Could you check a few things on this model? Use its own coordinates, in mm. A direction names the side the tool comes from. Round coordinates to 2 decimals unless told otherwise and drop trailing zeros. Order: outer loops, then holes, each group sorted by start corner. A loop starts at its lowest first (then second) coordinate and runs counter-clockwise, first axis right, second up. Notation, with made-up numbers: (85, 88) -> (110, 88) arc R26 cw to (110, 104) -> close; hole circle Ø5 at (-1.5, -28). An arc over 180 degrees is marked (long way). One line per question, with ' | ' between items.
```python
from build123d import *

# Parameters (mm, degrees)
CROQUIS1_R              = 2
SALIENTE_EXTRUIR1_DEPTH = 13
CROQUIS2_W              = 22
CROQUIS2_H              = 25
CORTAR_EXTRUIR1_DEPTH   = 52.980765673
REDONDEO1_R             = 5


with BuildPart() as part:
    # Croquis1 → Saliente-Extruir1 (new body)
    with BuildSketch(Plane.XY):
        with BuildLine():
            Line((5, 0), (33, 0))
            ThreePointArc((33, 0), (36.535533906, 1.464466094), (38, 5))
            ThreePointArc((38, 5), (35.19797288, 16.5), (38, 28))
            ThreePointArc((38, 28), (36.535533906, 31.535533906), (33, 33))
            Line((33, 33), (5, 33))
            ThreePointArc((5, 33), (1.464466094, 31.535533906), (0, 28))
            ThreePointArc((0, 28), (2.80202712, 16.5), (0, 5))
            ThreePointArc((0, 5), (1.464466094, 1.464466094), (5, 0))
        make_face()
        with Locations(Location((4, 4.75, 0), (0, 0, 180))):
            Circle(CROQUIS1_R, mode=Mode.SUBTRACT)
        with Locations(Location((34, 4.75, 0), (0, 0, 180))):
            Circle(CROQUIS1_R, mode=Mode.SUBTRACT)
        with Locations(Location((34, 28.25, 0), (0, 0, 180))):
            Circle(CROQUIS1_R, mode=Mode.SUBTRACT)
        with Locations(Location((4, 28.25, 0), (0, 0, 180))):
            Circle(CROQUIS1_R, mode=Mode.SUBTRACT)
    extrude(amount=SALIENTE_EXTRUIR1_DEPTH)

    # Croquis2 → Cortar-Extruir1 (cut, through all)
    with BuildSketch(Plane(origin=(0, 0, 0), x_dir=(-1, 0, 0), z_dir=(0, 0, -1))):
        with Locations((-19, 16.5)):
            Rectangle(CROQUIS2_W, CROQUIS2_H)
    extrude(amount=-CORTAR_EXTRUIR1_DEPTH, mode=Mode.SUBTRACT)

    # Redondeo1
    redondeo1_edges = [part.edges().sort_by_distance(p)[0] for p in [
        (8, 4, 6.5),
        (30, 4, 6.5),
        (30, 29, 6.5),
        (8, 29, 6.5),
    ]]
    fillet(redondeo1_edges, radius=REDONDEO1_R)


solid = part.part
```
1. I need wall thicknesses on probe 1 along Y at (x, z) = (24, 5); probe 2 along Y at (x, z) = (4, 6.5); probe 3 along X at (y, z) = (4.75, 8.5). Which ranges of each line are inside material? Lowest first, please.
From the geometry:
probe 1: y = 0 to 4, 29 to 33 | probe 2: y = 0.1 to 2.75, 6.75 to 26.25, 30.25 to 32.9 | probe 3: x = 0.01 to 2, 6 to 10.37, 27.63 to 32, 36 to 37.99
2. I'm going to push flat-ended pins straight in: pin 1 (3.5 mm diameter, centred on x = 4, y = 4.75, fed in from +Z); pin 2 (3 mm diameter, centred on y = 22, z = 7, fed in from +X); pin 3 (1.5 mm diameter, centred on y = 21, z = 9, fed in from +X); pin 4 (6.5 mm diameter, centred on y = 15, z = 8, fed in from -X). Where does each tip first touch, or does it pass through?
From the geometry:
pin 1: passes through | pin 2: stops at x = 36.2 | pin 3: stops at x = 35.76 | pin 4: stops at x = 2.35
3. I want a section at A-A on x = 9. List the corners of the cut face in (y, z) for me.
From the geometry:
outline: (0, 0) -> (6, 0) -> (6, 13) -> (0, 13) -> close; (27, 0) -> (33, 0) -> (33, 13) -> (27, 13) -> close
4. If we mould it in two halves opening along Y, with no side actions, what happens to faces 1 (the face through (6, 17, 0)), 2 (the face through (8, 16, 6)), 3 (the face through (19, 0, 6))? For each: pulls with the +Y half, pulls with the -Y half, needs draft (parallel to the pull), parting line crosses it, or undercut.
From the geometry:
face 1: needs draft | face 2: undercut | face 3: pulls with the -Y half
5. I want a section at D-D on x = 4. List the corners of the cut face in (y, z) for me, and give its area (3 significant figures).
From the geometry:
outline: (0.1, 0) -> (2.75, 0) -> (2.75, 13) -> (0.1, 13) -> close; (6.75, 0) -> (26.25, 0) -> (26.25, 13) -> (6.75, 13) -> close; (30.25, 0) -> (32.9, 0) -> (32.9, 13) -> (30.25, 13) -> close | area: 322 mm²
6. On a 3-axis mill with a long thin cutter (end or side, diameter ignored), from which of +Z, -Z, +X, -X, +Y, -Y can I reach the whole of each face in a straight line? I mean faces 4 (the face through (35.2, 16.3, 6.4)), 5 (the face through (30, 16, 6)). Say none if no direction works.
From the geometry:
face 4: +Z, -Z, +X | face 5: +Z, -Z
7. I want a section at B-B on z = 6.5. List the corners of the cut face in (x, y) for me, and give its area (3 significant figures).
From the geometry:
outline: (0, 5) arc R5 ccw to (5, 0) -> (33, 0) arc R5 ccw to (38, 5) arc R25 cw to (38, 28) arc R5 ccw to (33, 33) -> (5, 33) arc R5 ccw to (0, 28) arc R25 cw to start; hole circle Ø4 at (4, 4.75); hole circle Ø4 at (4, 28.25); hole (8, 9) arc R5 ccw to (13, 4) -> (25, 4) arc R5 ccw to (30, 9) -> (30, 24) arc R5 ccw to (25, 29) -> (13, 29) arc R5 ccw to (8, 24) -> close; hole circle Ø4 at (34, 4.75); hole circle Ø4 at (34, 28.25) | area: 567 mm²
8. I want a section at C-C on y = 19.5. List the corners of the cut face in (x, z) for me.
From the geometry:
outline: (2.62, 0) -> (8, 0) -> (8, 13) -> (2.62, 13) -> close; (30, 0) -> (35.38, 0) -> (35.38, 13) -> (30, 13) -> close
